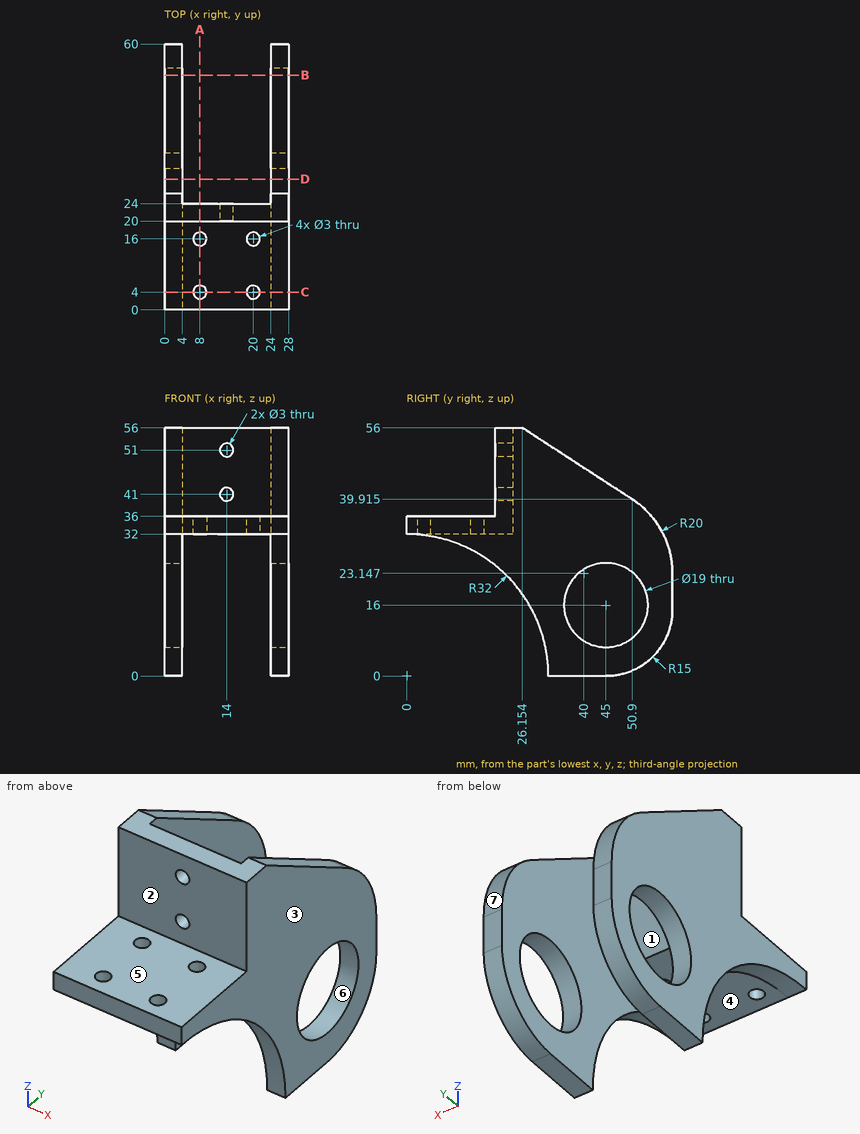
Print and shaded views of the part. All mm, measured from the part's lowest x, y and z. A direction names the side the tool comes from. Coordinates: 2 decimals unless noted, no trailing zeros. Loops run counter-clockwise (first coordinate to the right, second up) from the corner with the lowest first, then second, coordinate; pieces in that order, holes last. Notation, with made-up numbers: M 89,-25.75 L 148,-25.75 A16 cw 148,-17.75 Z; hole C -25.5,-29 d5. An arc over 180 degrees is marked long. Use a Markdown table: item, result. Add a question column.
Q1. Cut at A-A (x = 8). Write the cut outline in (y, z).
Q2. Probe L1, parallel to Y at x = 8, z = 34.5; L2, parallel to Z at x = 14, y = 21.45; L3, parallel to X at y = 34, z = 3. List the from-to ranges inside material, lowest first.
Q3. Pin check, flat tips, straight feed: P1, Ø10, axis at x = 19, y = 9.5, coming from the +Z side; P2, Ø10, axis at x = 19, z = 44, coming from the -Y side; P3, Ø1, axis at x = 12, y = 21, coming from the -Z side. Stop position of each tip, or through.
Q4. Mould opens along Y. For the marked faces 5, 6 and 7 say: +Y half, -Y half, draft (parallel to the pull), parting line (faces both ways), or undercut.
Q5. Cut at C-C (y = 4). Write the cut outline in (x, z).
Q6. Cut at B-B (y = 53). Write the cut outline in (x, z) (1 decimal), and give its area (3 significant figures).
Q7. Cut at D-D (y = 29.5). Write the cut outline in (x, z) (1 decimal).
Q8. Which spindle directions (+Z, -Z, +X, -X, +Y, -Y) get a long thin tool onto all of the face, cutting with end or side? Do the marked faces 1, 2, 3 and 4. Say none if no direction does.
Worked out:
| question | item | result |
|---|---|---|
| 1 | outline | M 0,32 L 2.5,32 L 2.5,36 L 0,36 Z; M 5.5,32 L 14.5,32 L 14.5,36 L 5.5,36 Z; M 17.5,32 L 24,32 L 24,56 L 20,56 L 20,36 L 17.5,36 Z |
| 2 | L1 | y = 0 to 2.5, 5.5 to 14.5, 17.5 to 24 |
| 2 | L2 | z = 32 to 39.5, 42.5 to 49.5, 52.5 to 56 |
| 2 | L3 | x = 0 to 4, 24 to 28 |
| 3 | P1 | stops at z = 36 |
| 3 | P2 | stops at y = 20 |
| 3 | P3 | stops at z = 32 |
| 4 | face 5 | draft |
| 4 | face 6 | undercut |
| 4 | face 7 | +Y half |
| 5 | outline | M 0,31.75 L 4,31.75 L 4,32 L 6.5,32 L 6.5,36 L 0,36 Z; M 9.5,32 L 18.5,32 L 18.5,36 L 9.5,36 Z; M 21.5,32 L 24,32 L 24,31.75 L 28,31.75 L 28,36 L 21.5,36 Z |
| 6 | outline | M 0,2.3 L 4,2.3 L 4,10.9 L 0,10.9 Z; M 0,21.1 L 4,21.1 L 4,38.3 L 0,38.3 Z; M 24,2.3 L 28,2.3 L 28,10.9 L 24,10.9 Z; M 24,21.1 L 28,21.1 L 28,38.3 L 24,38.3 Z |
| 6 | area | 206 mm2 |
| 7 | outline | M 0,12.4 L 4,12.4 L 4,53.8 L 0,53.8 Z; M 24,12.4 L 28,12.4 L 28,53.8 L 24,53.8 Z |
| 8 | face 1 | +Z, -Z, +Y |
| 8 | face 2 | +Z, +X, -X, -Y |
| 8 | face 3 | +Z, -Z, +X, +Y, -Y |
| 8 | face 4 | -Z, +Y, -Y |
